The listing builds one solid part. Answer for the finished solid, in the listing's coordinates (mm). Round coordinates to 2 decimals unless told otherwise and drop trailing zeros. Order: outer loops, then holes, each group sorted by start corner. A loop starts at its lowest first (then second) coordinate and runs counter-clockwise, first axis right, second up. Notation, with made-up numbers: (7.25, -7) -> (40.25, -7) arc R26 cw to (40.25, 29) -> close; hole circle Ø11 at (61.25, 75.25). An arc over 180 degrees is marked (long way). Answer in a Markdown table with one row per item. Add a question column.
```python
from build123d import *

# Parameters (mm, degrees)
SKETCH_1_W      = 2.85
SKETCH_1_H      = 2.85
EXTRUDE_1_DEPTH = 3
FILLET_1_R      = 0.5


with BuildPart() as part:
    # Эскиз1 → Бобышка-Вытянуть1 (new body)
    with BuildSketch(Plane(origin=(0, 0, 0), x_dir=(1, 0, 0), z_dir=(0, 1, 0))):
        Polygon((-52, 0), (52, 0), (52, 7), (55, 7), (55, 22), (45, 22), (45, 35), (-45, 35), (-45, 22), (-55, 22), (-55, 7), (-52, 7), align=None)
        with Locations((40.5, 3.5)):
            Rectangle(SKETCH_1_W, SKETCH_1_H, mode=Mode.SUBTRACT)
        with Locations((-40.5, 3.5)):
            Rectangle(SKETCH_1_W, SKETCH_1_H, mode=Mode.SUBTRACT)
    extrude(amount=EXTRUDE_1_DEPTH)

    # Скругление1
    fillet_1_edges = [part.edges().sort_by_distance(p)[0] for p in [
        (-55, 1.5, -7),
        (-55, 1.5, -22),
        (55, 1.5, -22),
        (55, 1.5, -7),
    ]]
    fillet(fillet_1_edges, radius=FILLET_1_R)


solid = part.part
```
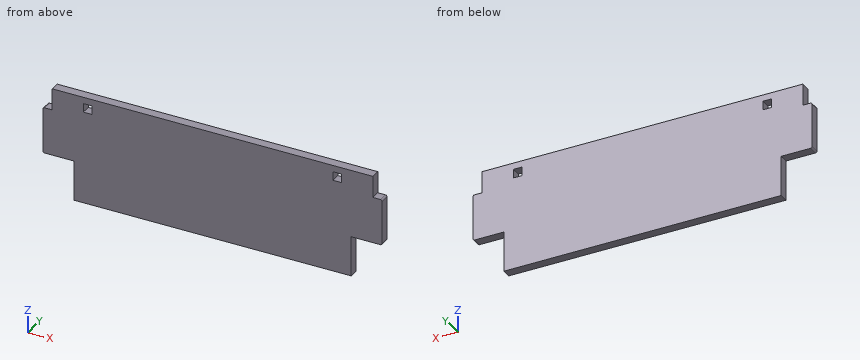
Item 1: The part is cut by section C-C, the plane z = -25.5. Give the vertices of the cut face in (x, y), and give its area (3 significant figures).
Item 2: Flat-ended cylindrical pins translate along their axes: P1, Ø0.9, axis at y = 1.5, z = -4, coming from the -X side; P2, Ø1.5, axis at y = 1.5, z = -31, coming from the -X side; P3, Ø1.5, axis at x = 49.5, y = 2, coming from the -Z side. Find the tip coordinate at first contact, or state that the pin passes through.
Item 3: The part is cut by section A-A, the plane z = -4. Give the vertices of the cut face in (x, y) (3 decimals), and give its area (3 significant figures).
Item 4: The part is cut by section B-B, the plane y = 1.55. Give the vertices of the cut face in (x, z) (3 decimals), and give its area (3 significant figures).
Item 5: Find the intervals of material crossed by probe 1 along Z at (x, y) = (39.5, 1.55) (3 decimals); probe 2 along X at (y, z) = (2.7, -33); probe 3 along Z at (x, y) = (-47, 0.65), in increasing order. Write a range as [from, to].
Resolved:
| question | item | result |
|---|---|---|
| 1 | outline | (-45, 0) -> (45, 0) -> (45, 3) -> (-45, 3) -> close |
| 1 | area | 270 mm2 |
| 2 | P1 | x = -52 |
| 2 | P2 | x = -45 |
| 2 | P3 | z = -22 |
| 3 | outline | (-52, 0) -> (-41.925, 0) -> (-41.925, 3) -> (-52, 3) -> close; (-39.075, 0) -> (39.075, 0) -> (39.075, 3) -> (-39.075, 3) -> close; (41.925, 0) -> (52, 0) -> (52, 3) -> (41.925, 3) -> close |
| 3 | area | 295 mm2 |
| 4 | outline | (-55, -21.5) arc R0.5 ccw to (-54.5, -22) -> (-45, -22) -> (-45, -35) -> (45, -35) -> (45, -22) -> (54.5, -22) arc R0.5 ccw to (55, -21.5) -> (55, -7.5) arc R0.5 ccw to (54.5, -7) -> (52, -7) -> (52, 0) -> (-52, 0) -> (-52, -7) -> (-54.5, -7) arc R0.5 ccw to (-55, -7.5) -> close; hole (-41.925, -4.925) -> (-39.075, -4.925) -> (-39.075, -2.075) -> (-41.925, -2.075) -> close; hole (39.075, -4.925) -> (41.925, -4.925) -> (41.925, -2.075) -> (39.075, -2.075) -> close |
| 4 | area | 3,530 mm2 |
| 5 | probe 1 | [-35, -4.925], [-2.075, 0] |
| 5 | probe 2 | [-45, 45] |
| 5 | probe 3 | [-22, 0] |
